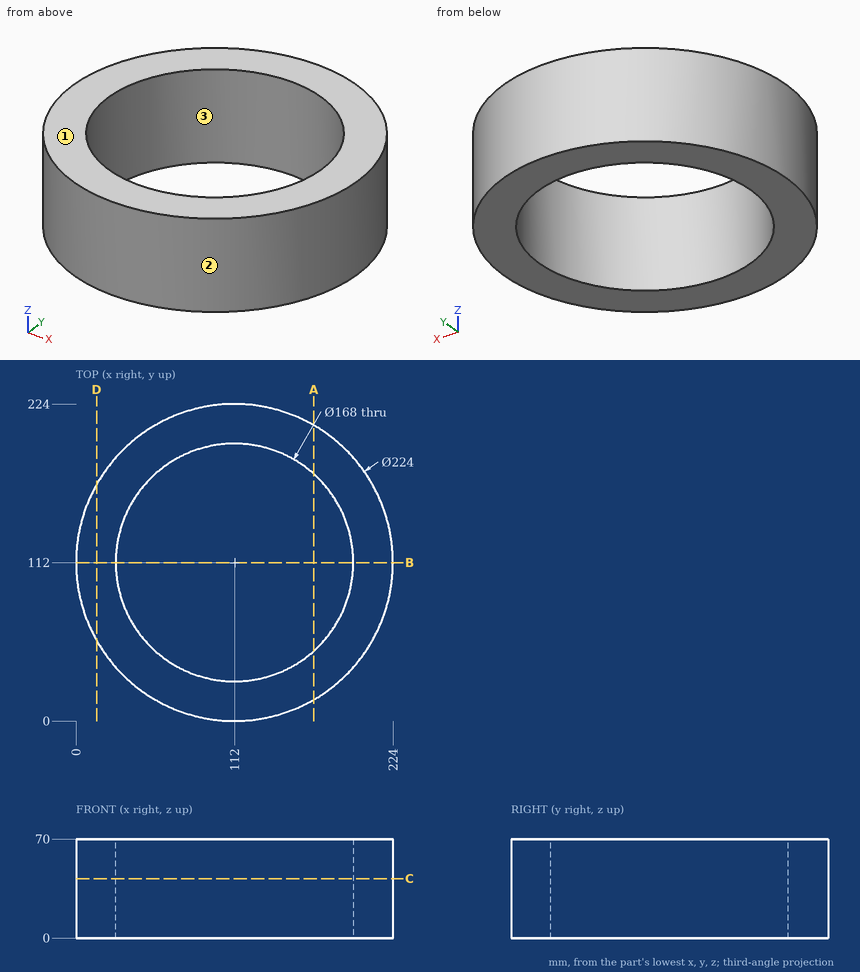
Drawing for the job (mm, zero at the part's lowest x, y, z). Give positions to 0.01 mm unless a question says otherwise; leave off trailing zeros. Loops run counter-clockwise (first coordinate to the right, second up) from the corner with the lowest first, then second, coordinate; pieces in that order, holes last.
(1) Band-saw the part on B-B (y = 112). Write the cut outline in (x, z), and give its area (3 significant figures).
Return value:
outline: (0, 0) - (28, 0) - (28, 70) - (0, 70) - close; (196, 0) - (224, 0) - (224, 70) - (196, 70) - close
area: 3,920 mm2
(2) Band-saw the part on D-D (x = 14.5). Write the cut outline in (y, z), and give its area (3 significant figures).
Return value:
outline: (56.88, 0) - (167.12, 0) - (167.12, 70) - (56.88, 70) - close
area: 7,720 mm2
(3) Drill centre lines: line 1 along Y through (x, z) = (112, 36); line 2 along Y through (x, z) = (137.5, 41); line 3 along X through (y, z) = (125, 41). Where is each one in solid material? Low to high.
Return value:
line 1: y = 0 to 28, 196 to 224
line 2: y = 2.94 to 31.96, 192.04 to 221.06
line 3: x = 0.76 to 29.01, 194.99 to 223.24
(4) Band-saw the part on A-A (x = 168). Write the cut outline in (y, z), and give its area (3 significant figures).
Return value:
outline: (15.01, 0) - (49.39, 0) - (49.39, 70) - (15.01, 70) - close; (174.61, 0) - (208.99, 0) - (208.99, 70) - (174.61, 70) - close
area: 4,810 mm2
(5) Pull direction X, two halves, no side cores. Call the marked faces 1, 2 and 3: pulls with the +X half, pulls with the -X half, needs draft (parallel to the pull), parting line crosses it, or undercut.
Return value:
face 1: needs draft
face 2: parting line crosses it
face 3: undercut
(6) Pin check, flat tips, straight feed: pin 1 (3 mm diameter, centred on y = 27.5, z = 31, fed in from -X); pin 2 (5 mm diameter, centred on y = 36, z = 24.5, fed in from -X); pin 3 (1.5 mm diameter, centred on y = 49.5, z = 38, fed in from -X). Stop position of each tip, or through.
Return value:
pin 1: stops at x = 36.8
pin 2: stops at x = 27.49
pin 3: stops at x = 18.56
(7) Band-saw the part on C-C (z = 42). Write the cut outline in (x, y).
Return value:
outline: circle Ø224 at (112, 112); hole circle Ø168 at (112, 112)
